Answer from the drawing. Dimensions are ordinates in mm from the lowest x, y and z of the part. A direction names the side the tool comes from. Coordinates: 2 decimals unless noted, no trailing zeros. Order: outer loops, then holes, each group sorted by start corner. A loop starts at its lowest first (then second) coordinate and runs counter-clockwise, first axis right, second up. Notation, with made-up numbers: (0.25, 1) -> (13.25, 1) arc R16 cw to (13.25, 14) -> close; hole circle Ø2 at (86, 48). An arc over 180 degrees is marked (long way). Answer in a Markdown table with one row per item.
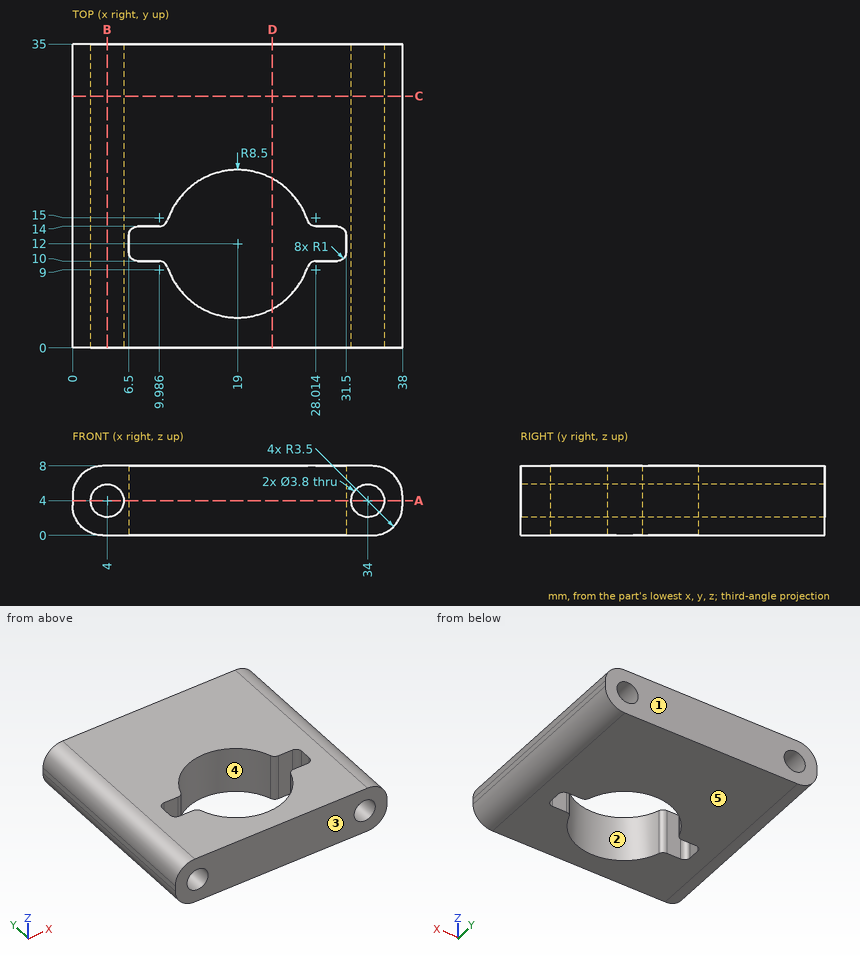
Q1. For a pull along Y with two mould halves and no side action, classify the marked faces 3, 4 and 5 as pulls with the +Y half, pulls with the -Y half, needs draft (parallel to the pull), parting line crosses it, or undercut.
Outcome:
| item | result |
|---|---|
| face 3 | pulls with the -Y half |
| face 4 | undercut |
| face 5 | needs draft |
Q2. Consider line 1 (Z direction, x = 4, y = 24); line 2 (Y direction, x = 29.5, z = 5); line 3 (X direction, y = 13.5, z = 3.5). Determine where each line is inside the solid, lowest interval first.
Outcome:
| item | result |
|---|---|
| line 1 | 0 to 2.1, 5.9 to 8 |
| line 2 | 0 to 10, 14 to 35 |
| line 3 | 0 to 2.17, 5.83 to 6.63, 31.37 to 32.17, 35.83 to 38 |
Q3. The part is cut by section D-D (x = 23). Write down the section's boundary in (y, z), then the cut area to 3 significant figures.
Outcome:
| item | result |
|---|---|
| outline | (0, 0) -> (4.5, 0) -> (4.5, 8) -> (0, 8) -> close; (19.5, 0) -> (35, 0) -> (35, 8) -> (19.5, 8) -> close |
| area | 160 mm² |
Q4. Given pin 1 (1 mm diameter, centred on y = 12, z = 5.5, fed in from +X); pin 2 (1 mm diameter, centred on y = 12.5, z = 2.5, fed in from -X); pin 3 (12 mm diameter, centred on x = 5.5, y = 8, fed in from -Z); pin 4 (2 mm diameter, centred on y = 22, z = 6.5, fed in from +X), each flat-ended and moving along its own axis, determine where each tip first touches the part or whether it passes through.
Outcome:
| item | result |
|---|---|
| pin 1 | x = 37.96 |
| pin 2 | x = 0.04 |
| pin 3 | z = 0 |
| pin 4 | x = 37.85 |
Q5. For the marked faces 1 and 2, determine the directions among +Z, -Z, +X, -X, +Y, -Y from which every point of the face is accessible in a straight line to the end or side of a thin tool.
Outcome:
| item | result |
|---|---|
| face 1 | +Z, -Z, +X, -X, +Y |
| face 2 | +Z, -Z |
Q6. The part is cut by section B-B (x = 4). Write down the section's boundary in (y, z).
Outcome:
| item | result |
|---|---|
| outline | (0, 0) -> (35, 0) -> (35, 2.1) -> (0, 2.1) -> close; (0, 5.9) -> (35, 5.9) -> (35, 8) -> (0, 8) -> close |
Q7. The part is cut by section A-A (z = 4). Write down the section's boundary in (x, y) (3 decimals).
Outcome:
| item | result |
|---|---|
| outline | (0, 0) -> (2.1, 0) -> (2.1, 35) -> (0, 35) -> close; (5.9, 0) -> (32.1, 0) -> (32.1, 35) -> (5.9, 35) -> close; (35.9, 0) -> (38, 0) -> (38, 35) -> (35.9, 35) -> close; hole (6.5, 11) arc R1 ccw to (7.5, 10) -> (9.986, 10) arc R1 cw to (10.935, 9.316) arc R8.5 ccw to (27.065, 9.316) arc R1 cw to (28.014, 10) -> (30.5, 10) arc R1 ccw to (31.5, 11) -> (31.5, 13) arc R1 ccw to (30.5, 14) -> (28.014, 14) arc R1 cw to (27.065, 14.684) arc R8.5 ccw to (10.935, 14.684) arc R1 cw to (9.986, 14) -> (7.5, 14) arc R1 ccw to (6.5, 13) -> close |
Q8. The part is cut by section C-C (y = 29). Write down the section's boundary in (x, z), then the cut area to 3 significant figures.
Outcome:
| item | result |
|---|---|
| outline | (0, 3.5) arc R3.5 ccw to (3.5, 0) -> (34.5, 0) arc R3.5 ccw to (38, 3.5) -> (38, 4.5) arc R3.5 ccw to (34.5, 8) -> (3.5, 8) arc R3.5 ccw to (0, 4.5) -> close; hole circle Ø3.8 at (4, 4); hole circle Ø3.8 at (34, 4) |
| area | 271 mm² |
